Read the model definition and answer for the solid it produces. Units are mm, in the model's axes. Face numbers are marked on the shaded views. A direction names the side the tool comes from. Give positions to 0.01 mm unless a question says otherwise; leave off trailing zeros. Loops run counter-clockwise (first coordinate to the right, second up) from the corner with the lowest first, then second, coordinate; pieces in that order, holes last.
(1) Find section D-D, the plane y = 123. Write down the section's boundary in (x, z) (1 decimal).
(2) Which of the six approach directions +Z, -Z, +X, -X, +Y, -Y give full straight-line access (tool end or side, diameter ignored) to the marked faces 1 and 2?
(3) Straight lines are drawn through the part: probe 1 along X at (y, z) = (88, 0) (3 decimals); probe 2 along X at (y, z) = (128, 0); probe 3 along Y at (x, z) = (8.5, -3.5) (3 decimals). For each, find the intervals that lie inside material, in ascending order.
(4) Find section C-C, the plane y = 36.5. Write down the section's boundary in (x, z) (3 decimals).
(5) Each of these flat-tipped pins is pushed along its axis until it touches: P1, Ø8, axis at y = 99.5, z = -8.5, coming from the +X side; P2, Ø13.5, axis at x = 3, z = 1.5, coming from the -Y side (3 decimals); P3, Ø18.5, axis at x = 0, z = 0, coming from the +Y side; P4, Ø8.5, axis at x = 0, z = 0, coming from the +Y side. Where does it stop, or does it pass through?
(6) Determine the mould class of the marked faces 3 and 4 for opening direction Z: pulls with the +Z half, pulls with the -Z half, needs draft (parallel to the pull), parting line crosses it, or undercut.
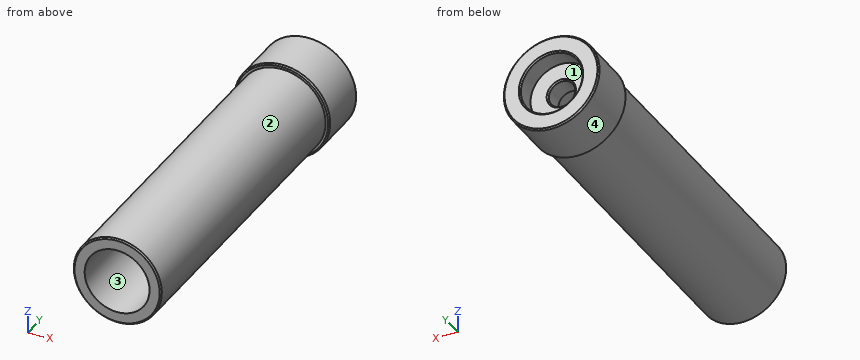
```python
from build123d import *

# Parameters (mm, degrees)
SKETCH1_R                    = 15.875
BOSS_EXTRUDE1_DEPTH          = 114.3
SKETCH2_R                    = 17.272
BOSS_EXTRUDE2_DEPTH          = 19.05
SKETCH10_R                   = 11.1125
CUT_EXTRUDE1_DEPTH           = 7.1628
F_3_8_0_375_DIAMETER_HOLE1_D = 9.525
SKETCH15_R                   = 11.7078125
CUT_EXTRUDE3_DEPTH           = 111.125
SKETCH16_R                   = 8.334375
CUT_EXTRUDE4_DEPTH           = 7.9375
CHAMFER2_SIZE                = 0.508


with BuildPart() as part:
    # Sketch1 → Boss-Extrude1 (new body)
    with BuildSketch(Plane(origin=(0, 0, 0), x_dir=(1, 0, 0), z_dir=(0, 1, 0))):
        with Locations(Location((0, 0, 0), (0, 0, 270))):
            Circle(SKETCH1_R)
    extrude(amount=BOSS_EXTRUDE1_DEPTH)

    # Sketch2 → Boss-Extrude2 (add)
    with BuildSketch(Plane(origin=(0, 114.3, 0), x_dir=(1, 0, 0), z_dir=(0, 1, 0))):
        with Locations(Location((0, 0, 0), (0, 0, 90))):
            Circle(SKETCH2_R)
    extrude(amount=BOSS_EXTRUDE2_DEPTH)

    # Sketch10 → Cut-Extrude1 (cut)
    with BuildSketch(Plane(origin=(0, 133.35, 0), x_dir=(1, 0, 0), z_dir=(0, 1, 0))):
        with Locations(Location((0, 0, 0), (0, 0, 270))):
            Circle(SKETCH10_R)
    extrude(amount=-CUT_EXTRUDE1_DEPTH, mode=Mode.SUBTRACT)

    # 3/8 (0.375) Diameter Hole1 (through all)
    with Locations(Plane(origin=(0, 126.1872, 0), x_dir=(1, 0, 0), z_dir=(0, 1, 0))):
        with Locations((0, 0)):
            Hole(F_3_8_0_375_DIAMETER_HOLE1_D / 2)

    # Sketch15 → Cut-Extrude3 (cut)
    with BuildSketch(Plane.XZ):
        with Locations(Location((0, 0, 0), (0, 0, 270))):
            Circle(SKETCH15_R)
    extrude(amount=-CUT_EXTRUDE3_DEPTH, mode=Mode.SUBTRACT)

    # Sketch16 → Cut-Extrude4 (cut)
    with BuildSketch(Plane.XZ.offset(-111.125)):
        with Locations(Location((0, 0, 0), (0, 0, 270))):
            Circle(SKETCH16_R)
    extrude(amount=-CUT_EXTRUDE4_DEPTH, mode=Mode.SUBTRACT)

    # Chamfer2
    chamfer2_edges = [part.edges().sort_by_distance(p)[0] for p in [
        (0, 133.35, -11.1125),
        (4.7625, 126.1872, 0),
        (0, 0, -15.875),
        (0, 114.3, 17.272),
        (0, 133.35, 17.272),
    ]]
    chamfer(chamfer2_edges, length=CHAMFER2_SIZE)


solid = part.part
```
Entries:
1. outline: circle Ø34.5 at (0, 0); hole circle Ø9.5 at (0, 0)
2. face 1: +Y
2. face 2: -Y
3. probe 1: x = -15.875 to -11.708, 11.708 to 15.875
3. probe 2: x = -17.27 to -11.11, 11.11 to 17.27
3. probe 3: y = 111.125 to 126.187
4. outline: circle Ø31.75 at (0, 0); hole circle Ø23.416 at (0, 0)
5. P1: stops at x = 15.22
5. P2: stops at y = 111.125
5. P3: stops at y = 126.19
5. P4: passes through
6. face 3: undercut
6. face 4: parting line crosses it
